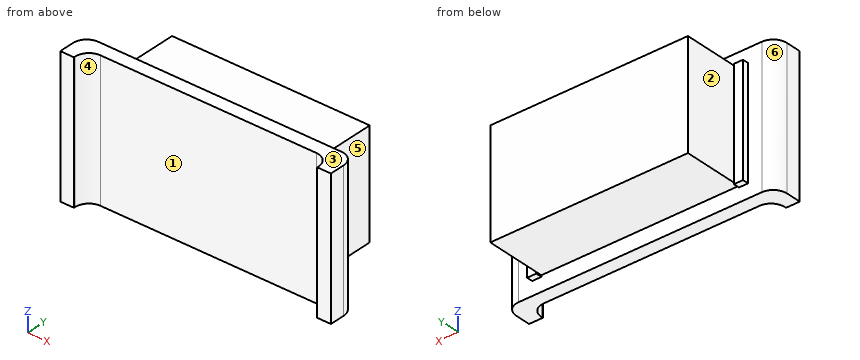
from build123d import *

# Parameters (mm, degrees)
ESQUISSE2_W              = 160
ESQUISSE2_H              = 90
EXTRUSION1_DEPTH         = 9
ESQUISSE1_W              = 130
ESQUISSE1_H              = 70
BEURRE_AVEC_MARGES_DEPTH = 40
ESQUISSE4_W              = 6
ESQUISSE4_H              = 72
EXTRUSION3_DEPTH         = 4
ESQUISSE6_W              = 9
ESQUISSE6_H              = 90
EXTRUSION4_DEPTH         = 19
CONG_1_R                 = 9


with BuildPart() as part:
    # Esquisse2 → Extrusion1 (new body)
    with BuildSketch(Plane(origin=(0, 0, 0), x_dir=(1, 0, 0), z_dir=(0, 1, 0))):
        with Locations((18.862465753, -11.339726027)):
            Rectangle(ESQUISSE2_W, ESQUISSE2_H)
    extrude(amount=-EXTRUSION1_DEPTH)

    # Esquisse1 → Beurre (avec marges) (add)
    with BuildSketch(Plane(origin=(0, 0, 0), x_dir=(1, 0, 0), z_dir=(0, 1, 0))):
        with Locations((18.862465753, -11.339726027)):
            Rectangle(ESQUISSE1_W, ESQUISSE1_H)
    extrude(amount=BEURRE_AVEC_MARGES_DEPTH)

    # Esquisse4 → Extrusion3 (add)
    with BuildSketch(Plane(origin=(0, 0, 0), x_dir=(1, 0, 0), z_dir=(0, 1, 0))):
        with Locations((-49.137534247, -11.339726027)):
            Rectangle(ESQUISSE4_W, ESQUISSE4_H)
        with Locations((86.862465753, -11.339726027)):
            Rectangle(ESQUISSE4_W, ESQUISSE4_H)
    extrude(amount=EXTRUSION3_DEPTH)

    # Esquisse6 → Extrusion4 (add)
    with BuildSketch(Plane(origin=(0, 0, 0), x_dir=(1, 0, 0), z_dir=(0, 1, 0))):
        with Locations((-65.637534247, -11.339726027)):
            Rectangle(ESQUISSE6_W, ESQUISSE6_H)
        with Locations((103.362465753, -11.339726027)):
            Rectangle(ESQUISSE6_W, ESQUISSE6_H)
    extrude(amount=-EXTRUSION4_DEPTH)

    # Congé1
    cong_1_edges = [part.edges().sort_by_distance(p)[0] for p in [
        (98.862465753, -9, 11.339726027),
        (-61.137534247, -9, 11.339726027),
        (107.862465753, 0, 11.339726027),
        (-70.137534247, 0, 11.339726027),
    ]]
    fillet(cong_1_edges, radius=CONG_1_R)


solid = part.part
The model under review builds one solid part; all positions refer to its coordinate system, in mm. Face numbers are marked on the shaded views. A direction names the side the tool comes from. Round coordinates to 2 decimals unless told otherwise and drop trailing zeros. Write each loop counter-clockwise with the first axis right and the second up, starting at its lowest first coordinate (ties: lowest second). Pieces come first, ordered by that corner, then holes. Notation, with made-up numbers: M 46,31.5 L 66,31.5 A15 cw 66,38.5 Z; hole C 31,75 d2. An arc over 180 degrees is marked long. Use a Markdown table: item, result. Add a question column.
Q1. We need section A-A, the plane x = -17. State the section outline as (y, z) points, plus the area to 3 significant figures.
Q2. The part is to be moulded in two halves that separate along X. For the marked faces 1, 2, 3 and 4, say which applies: pulls with the +X half, pulls with the -X half, needs draft (parallel to the pull), parting line crosses it, or undercut.
Q3. We need section D-D, the plane x = -58.5. State the section outline as (y, z) points, plus the area to 3 significant figures.
Q4. Insertion check: pin 1 (18 mm diameter, centred on y = 20.5, z = 0, fed in from +X); pin 2 (1.1 mm diameter, centred on y = 1, z = -24, fed in from +X); pin 3 (1.2 mm diameter, centred on x = 88, y = 2.5, fed in from -Z); pin 4 (3 mm diameter, centred on x = 13.5, z = -24, fed in from +Y). Each pin has a flat end and moves straight along its axis. Give the tip position at first contact, or say it passes through.
Q5. To check wall thickness, follow line 1 (Z direction, x = 5.5, y = 32.5); line 2 (X direction, y = 18.5, z = -23.5); line 3 (Y direction, x = 26, z = -9.5). State the ranges of each line that lie inside material, in increasing order.
Q6. We need section C-C, the plane y = 30.5. State the section outline as (x, z) points.
Q7. We need section B-B, the plane z = 17. State the section outline as (x, y) points.
Q8. Machinability: for the marked faces 5 and 6, which of the approach directions +Z, -Z, +X, -X, +Y, -Y give a long, thin tool a straight path to every point of the face, cutting with its end or side? Answer none if there is none.
Findings below:
| question | item | result |
|---|---|---|
| 1 | outline | M -9,-33.66 L 0,-33.66 L 0,-23.66 L 40,-23.66 L 40,46.34 L 0,46.34 L 0,56.34 L -9,56.34 Z |
| 1 | area | 3,610 mm² |
| 2 | face 1 | undercut |
| 2 | face 2 | pulls with the -X half |
| 2 | face 3 | needs draft |
| 2 | face 4 | undercut |
| 3 | outline | M -11.63,-33.66 L 0,-33.66 L 0,56.34 L -11.63,56.34 Z |
| 3 | area | 1,050 mm² |
| 4 | pin 1 | stops at x = 83.86 |
| 4 | pin 2 | stops at x = 89.86 |
| 4 | pin 3 | stops at z = -24.66 |
| 4 | pin 4 | stops at y = 40 |
| 5 | line 1 | z = -23.66 to 46.34 |
| 5 | line 2 | x = -46.14 to 83.86 |
| 5 | line 3 | y = -9 to 40 |
| 6 | outline | M -46.14,-23.66 L 83.86,-23.66 L 83.86,46.34 L -46.14,46.34 Z |
| 7 | outline | M -70.14,-19 L -61.14,-19 L -61.14,-18 A9 cw -52.14,-9 L 89.86,-9 A9 cw 98.86,-18 L 98.86,-19 L 107.86,-19 L 107.86,-9 A9 ccw 98.86,0 L 89.86,0 L 89.86,4 L 83.86,4 L 83.86,40 L -46.14,40 L -46.14,4 L -52.14,4 L -52.14,0 L -61.14,0 A9 ccw -70.14,-9 Z |
| 8 | face 5 | +Z, -Z, +X, +Y |
| 8 | face 6 | +Z, -Z, -X, +Y |
